Input: dimensioned drawing with shaded views. Units: mm. Origin: part minimum x, y, z. Round coordinates to 2 decimals unless told otherwise and drop trailing zeros. Use CSV: the item, a comma, the result in double quotes. Start each with the question number.
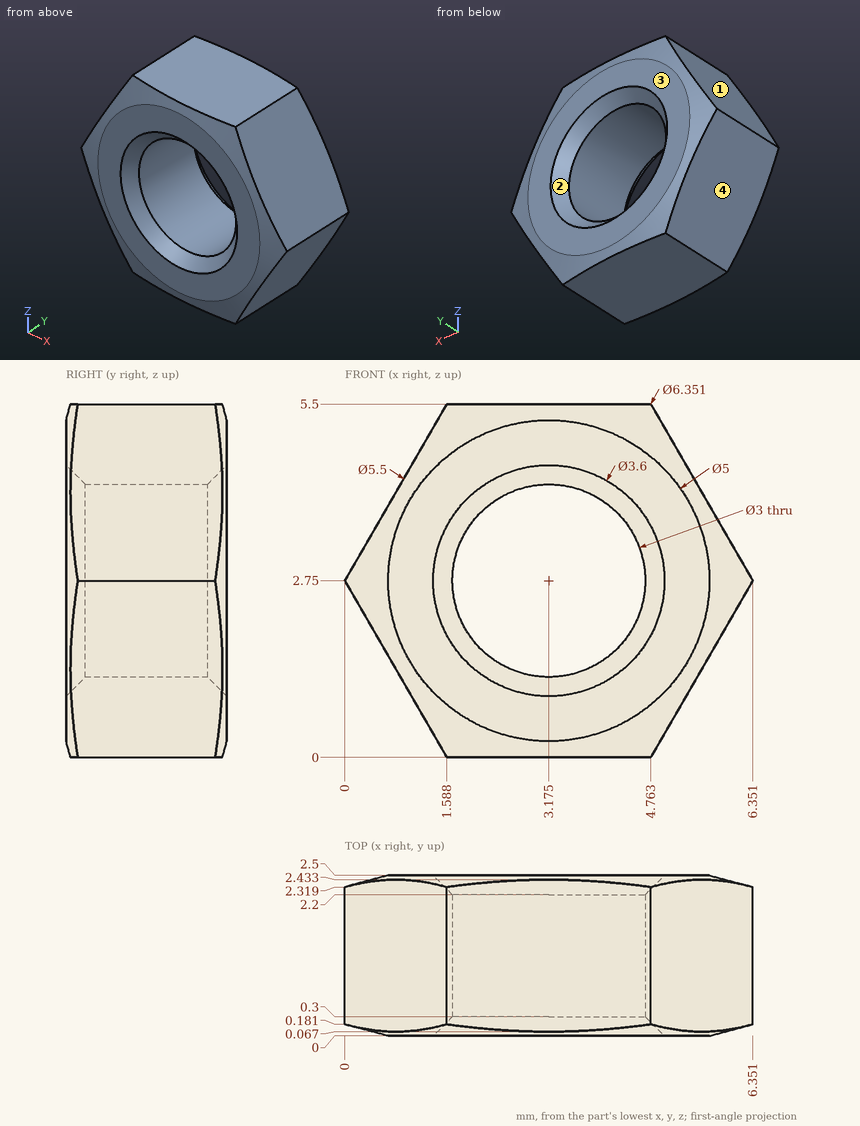
1. Line query: line 1 along Y through (x, z) = (1, 4); line 2 along X through (y, z) = (0.35, 1.9); line 3 along Z through (x, y) = (2, 1.75). Output: solid intervals per line, ascending.
2. Contact query for a flat-ended pin moving along its axis: P1, Ø3, axis at x = 3.5, z = 3, coming from the +Y side. Output: stop coordinate, or through.
3. Mould query, pull axis Z, two halves, no side actions, for the marked faces 1, 2, 3 and 4. Classes: +Z half, -Z half, draft (parallel to the pull), parting line (faces both ways), or undercut.
Values:
1,line 1,"y = 0 to 2.5"
1,line 2,"x = 0.49 to 1.94, 4.41 to 5.86"
1,line 3,"z = 0 to 1.82, 3.68 to 5.5"
2,P1,"stops at y = 2.5"
3,face 1,"+Z half"
3,face 2,"undercut"
3,face 3,"draft"
3,face 4,"-Z half"
